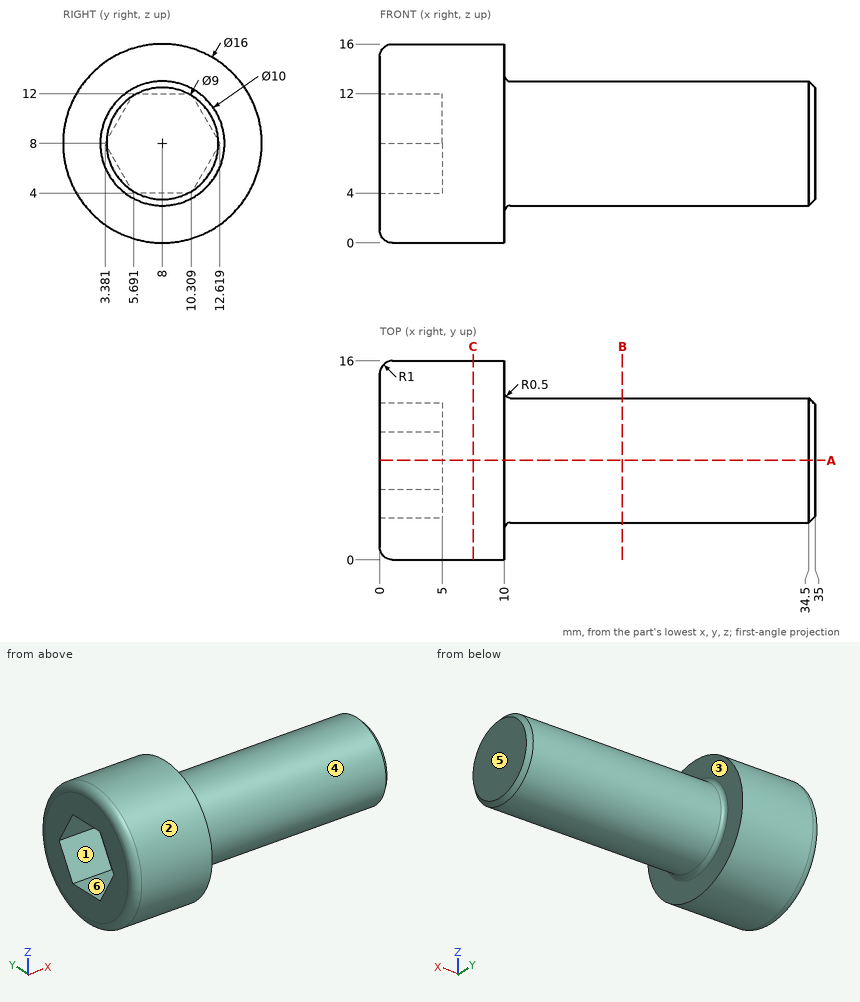
Can you work these out from the drawing? Everything is in mm from the part's minimum corner. A direction names the side the tool comes from. Coordinates: 2 decimals unless noted, no trailing zeros. Order: outer loops, then holes, each group sorted by start corner. A loop starts at its lowest first (then second) coordinate and runs counter-clockwise, first axis right, second up. Notation, with made-up numbers: M 15,12.5 L 26,12.5 A35 ccw 26,51.5 Z; hole C 74,-32.75 d7. An arc over 180 degrees is marked long. Answer as CSV lines item,"result". Start each with the question number.
1. We'd pull the mould along Z, two halves only. Please class the marked faces 1, 2 and 3: released by +Z, released by -Z, zero draft, split by the parting line, or undercut.
2. I want a section at C-C, the plane x = 7.5. Write out the boundary of the cut face in (y, z), and give its area (3 significant figures).
3. I want a section at B-B, the plane x = 19.5. Write out the boundary of the cut face in (y, z).
4. I want a section at A-A, the plane y = 8. Write out the boundary of the cut face in (x, z).
5. On a 3-axis mill with a long thin cutter (end or side, diameter ignored), from which of +Z, -Z, +X, -X, +Y, -Y can I reach the whole of each face in a straight line? I mean the marked faces 4, 5 and 6. Say none if no direction works.
6. I need wall thicknesses on line 1 (X direction, y = 10.5, z = 10); line 2 (X direction, y = 10.5, z = 2.75); line 3 (Z direction, x = 4.5, y = 9.25). Which ranges of each line are inside material? Lowest first, please. Write a range as [from, to].
7. For pin 1 (8 mm diameter, centred on x = 27.5, z = 6.5, fed in from +Y); pin 2 (4 mm diameter, centred on x = 27, y = 8.5, fed in from +Z); pin 3 (5 mm diameter, centred on y = 14, z = 4, fed in from +X), each with a flat end and sliding along its axis, tell me the tip position at first contact or that it passes through.
Recorded:
1,face 1,"undercut"
1,face 2,"split by the parting line"
1,face 3,"zero draft"
2,outline,"C 8,8 d16"
2,area,"201 mm2"
3,outline,"C 8,8 d10"
4,outline,"M 0,1 A1 ccw 1,0 L 10,0 L 10,2.5 A0.5 cw 10.5,3 L 34.5,3 L 35,3.5 L 35,12.5 L 34.5,13 L 10.5,13 A0.5 cw 10,13.5 L 10,16 L 1,16 A1 ccw 0,15 L 0,12 L 5,12 L 5,4 L 0,4 Z"
5,face 4,"+X"
5,face 5,"+Z, -Z, +X, +Y, -Y"
5,face 6,"-X"
6,line 1,"x = [5, 35]"
6,line 2,"x = [0, 10]"
6,line 3,"z = [0.1, 4], [12, 15.9]"
7,pin 1,"stops at y = 13"
7,pin 2,"stops at z = 13"
7,pin 3,"stops at x = 34.79"
